from build123d import *

# Parameters (mm, degrees)
SKETCH1_W                  = 140
SKETCH1_H                  = 20
F_8_2_8_2_DIAMETER_HOLE1_D = 8.2
HOLE1_D                    = 212
HOLE1_CBORE_D              = 240
HOLE1_CBORE_DEPTH          = 15
CHAMFER1_SIZE              = 1


with BuildPart() as part:
    # Sketch1 → Revolve1 (revolve)
    with BuildSketch(Plane.XZ, mode=Mode.PRIVATE) as revolve1_sk:
        with Locations((70, 10)):
            Rectangle(SKETCH1_W, SKETCH1_H)
    revolve(revolve1_sk.sketch.rotate(Axis((0, 0, 20), (0, 0, -1)), 180), axis=Axis((0, 0, 20), (0, 0, -1)))

    # Ø8.2 (8.2) Diameter Hole1 (through all)
    with Locations(Plane.XY.offset(20)):
        with Locations((49.748846207, 120.104339226), (120.104339226, 49.748846207), (120.104339226, -49.748846207), (49.748846207, -120.104339226), (-49.748846207, -120.104339226), (-120.104339226, -49.748846207), (-120.104339226, 49.748846207), (-49.748846207, 120.104339226)):
            Hole(F_8_2_8_2_DIAMETER_HOLE1_D / 2)

    # Hole1 (through all)
    with Locations(Plane.XY.offset(20)):
        with Locations((0, 0)):
            CounterBoreHole(HOLE1_D / 2, HOLE1_CBORE_D / 2, HOLE1_CBORE_DEPTH)

    # Chamfer1
    chamfer1_edges = [part.edges().sort_by_distance(p)[0] for p in [
        (140, 0, 0),
        (140, 0, 20),
        (-120, 0, 20),
        (106, 0, 0),
        (106, 0, 5),
    ]]
    chamfer(chamfer1_edges, length=CHAMFER1_SIZE)


solid = part.part
Read the model definition and answer for the solid it produces. Units are mm, in the model's axes. A direction names the side the tool comes from. Give positions to 0.01 mm unless a question says otherwise; leave off trailing zeros. Write each loop counter-clockwise with the first axis right and the second up, starting at its lowest first coordinate (ties: lowest second). Pieces come first, ordered by that corner, then holes. Notation, with made-up numbers: (19.25, -34.75) -> (30.25, -34.75) arc R22 ccw to (30.25, -12.75) -> close; hole circle Ø1 at (2.5, 47). An arc over 180 degrees is marked (long way). Answer as a JSON object with one key per item and string values. Group by question number.
1) Each of these flat-tipped pins is pushed along its axis until it touches: P1, Ø1, axis at x = -98, z = 10, coming from the -Y side; P2, Ø1.5, axis at x = -3.5, z = 11.5, coming from the -Y side; P3, Ø8, axis at x = -9, z = 7, coming from the +Y side. Where does it stop, or does it pass through?
2) Find section C-C (z = 15.75). Count the separate pieces of the cut face and the enclosed holes in it, and give its area (3 significant figures).
3) Consider L1, parallel to Y at x = 1, z = 6.75; L2, parallel to Y at x = 0, z = 2.3; L3, parallel to X at y = -52, z = 5.5. Determine where each line is inside the solid, lowest interval first. Write a range as from..to.
4) Find section A-A (x = 0). Write down the section's boundary in (y, z), and give its area (3 significant figures).
5) A tool of negligible diameter and unlimited length cuts with its end or side. For faces 4 (the cylindrical face through (-116.01, 49.93, 9.86)), 5 (the flat face through (-107.2, 0.6, 5)), from which of +Z, -Z, +X, -X, +Y, -Y can it reach the whole face along a straight path? Write none if from no direction.
6) The mould has two halves that part along Y. Classify faces 1 (the flat face through (-114, 42, 20)), 2 (the cylindrical face through (30.35, -136.67, 10.13)), 3 (the cylindrical face through (-48.86, -124.107, 9.86)): +Y half, -Y half, draft (parallel to the pull), parting line (faces both ways), or undercut.
Values follow:
{
 "1": {"P1": "stops at y = -100.47", "P2": "stops at y = -139.97", "P3": "stops at y = 139.91"},
 "2": {"separate pieces": "1", "enclosed holes": "9", "area": "15,900 mm2"},
 "3": {"L1": "y = -140..-120, 120..140", "L2": "y = -140..-106, 106..140", "L3": "x = -129.98..-123.53, -116.68..-108.15, 108.15..116.68, 123.53..129.98"},
 "4": {"outline": "(-140, 1) -> (-139, 0) -> (-107, 0) -> (-106, 1) -> (-106, 4) -> (-107, 5) -> (-120, 5) -> (-120, 19) -> (-121, 20) -> (-139, 20) -> (-140, 19) -> close; (106, 1) -> (107, 0) -> (139, 0) -> (140, 1) -> (140, 19) -> (139, 20) -> (121, 20) -> (120, 19) -> (120, 5) -> (107, 5) -> (106, 4) -> close", "area": "935 mm2"},
 "5": {"face 4": "+Z, -Z", "face 5": "+Z"},
 "6": {"face 1": "draft", "face 2": "parting line", "face 3": "undercut"}
}
